Could you check a few things on this model? Use its own coordinates, in mm. Face numbers are marked on the shaded views. A direction names the side the tool comes from. Round coordinates to 2 decimals unless told otherwise and drop trailing zeros. Loops run counter-clockwise (first coordinate to the right, second up) from the corner with the lowest first, then second, coordinate; pieces in that order, holes last. Notation, with made-up numbers: (46, 69.5) -> (84, 69.5) arc R21 cw to (84, 92.5) -> close; hole circle Ø6 at (-9.75, 55). An arc over 180 degrees is marked (long way). Write each question's results on one line, items separated by ' | '.
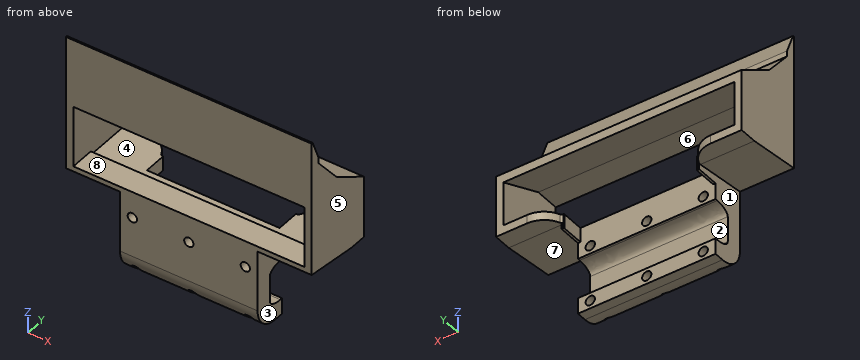
from build123d import *

# Parameters (mm, degrees)
RESSALTO_EXTRUS_O1_DEPTH = 30
CORTE_EXTRUS_O1_DEPTH    = 100
ESBO_O4_W                = 94
ESBO_O4_H                = 25
CORTE_EXTRUS_O2_DEPTH    = 10
ESBO_O5_W                = 94
ESBO_O5_H                = 18
CORTE_EXTRUS_O3_DEPTH    = 20
CORTE_EXTRUS_O7_START    = -3
CORTE_EXTRUS_O7_DEPTH    = 94
ESBO_O8_W                = 32
ESBO_O8_H                = 15
CORTE_EXTRUS_O8_DEPTH    = 56
ESBO_O9_W                = 16.5
ESBO_O9_H                = 8
CORTE_EXTRUS_O9_DEPTH    = 56
FILETE1_SIZE             = 3
FILETE1_SIZE_2           = 6
FILETE2_SIZE             = 3
FILETE2_SIZE_2           = 6
FILETE3_R                = 10
ESBO_O12_W               = 32
ESBO_O12_H               = 1
CORTE_EXTRUS_O12_DEPTH   = 68
CORTE_EXTRUS_O13_REACH   = 121.432
ESBO_O14_W               = 56
ESBO_O14_H               = 16
CORTE_EXTRUS_O14_DEPTH   = 138.840487586
ESBO_O16_R               = 1.9
CORTE_EXTRUS_O15_DEPTH   = 136.484316502
ESBO_O19_W               = 5.89
ESBO_O19_H               = 9.379485794
RESSALTO_EXTRUS_O4_DEPTH = 1
ESBO_O20_W               = 5.89
ESBO_O20_H               = 9.379485794
RESSALTO_EXTRUS_O5_DEPTH = 1
FILETE5_R                = 10
FILETE6_R                = 0.3
FILETE7_R                = 1
CORTE_EXTRUS_O17_DEPTH   = 22
CORTE_EXTRUS_O18_DEPTH   = 22
CORTE_EXTRUS_O19_DEPTH   = 124


with BuildPart() as part:
    # Esboço2 → Ressalto-extrusão1 (new body)
    with BuildSketch(Plane(origin=(0, 0, 0), x_dir=(1, 0, 0), z_dir=(0, 1, 0))):
        Polygon((0, 0), (0, 58), (22, 58), (22, 90), (78, 90), (78, 58), (100, 58), (100, 0), align=None)
    extrude(amount=RESSALTO_EXTRUS_O1_DEPTH)

    # Esboço3 → Corte-extrusão1 (cut)
    with BuildSketch(Plane(origin=(100, 0, 0), x_dir=(0, 0, -1), z_dir=(1, 0, 0))):
        Polygon((0, 0.6), (9.828405069, 4.570933406), (22.126818959, 14.890527965), (31.568264957, 30), (0, 30), align=None)
    extrude(amount=-CORTE_EXTRUS_O1_DEPTH, mode=Mode.SUBTRACT)

    # Esboço4 → Corte-extrusão2 (cut)
    with BuildSketch(Plane.XZ):
        with Locations((50, -40.5)):
            Rectangle(ESBO_O4_W, ESBO_O4_H)
    extrude(amount=-CORTE_EXTRUS_O2_DEPTH, mode=Mode.SUBTRACT)

    # Esboço5 → Corte-extrusão3 (cut)
    with BuildSketch(Plane(origin=(0, 30, 0), x_dir=(1, 0, 0), z_dir=(0, 1, 0))):
        with Locations((50, 45.5)):
            Rectangle(ESBO_O5_W, ESBO_O5_H)
    extrude(amount=-CORTE_EXTRUS_O3_DEPTH, mode=Mode.SUBTRACT)

    # Esboço7 → Corte-extrusão7 (cut)
    with BuildSketch(Plane(origin=(100, 0, 0), x_dir=(0, 0, -1), z_dir=(1, 0, 0)).offset(CORTE_EXTRUS_O7_START)):
        Polygon((28, 10), (36.5, 30), (36.5, 10), align=None)
    extrude(amount=-CORTE_EXTRUS_O7_DEPTH, mode=Mode.SUBTRACT)

    # Esboço8 → Corte-extrusão8 (cut)
    with BuildSketch(Plane(origin=(78, 0, 0), x_dir=(0, 0, -1), z_dir=(1, 0, 0))):
        with Locations((74, 22.5)):
            Rectangle(ESBO_O8_W, ESBO_O8_H)
    extrude(amount=-CORTE_EXTRUS_O8_DEPTH, mode=Mode.SUBTRACT)

    # Esboço9 → Corte-extrusão9 (cut)
    with BuildSketch(Plane(origin=(78, 0, 0), x_dir=(0, 0, -1), z_dir=(1, 0, 0))):
        with Locations((75.25, 11)):
            Rectangle(ESBO_O9_W, ESBO_O9_H)
    extrude(amount=-CORTE_EXTRUS_O9_DEPTH, mode=Mode.SUBTRACT)

    # Filete1
    # an asymmetric fillet: 6, 3 mm, written as the material it adds along each edge
    with BuildSketch(Plane(origin=(78, 7, -67), x_dir=(0, 0, -1), z_dir=(-1, 0, 0))) as filete1_piece_1:
        with BuildLine():
            Bezier((FILETE1_SIZE, 0), (0, 0), (0, -FILETE1_SIZE_2), weights=[1, 0.707106781, 1])
            Line((0, -FILETE1_SIZE_2), (0, 0))
            Line((0, 0), (FILETE1_SIZE, 0))
        make_face()
    extrude(amount=56)

    # Filete2
    # an asymmetric fillet: 6, 3 mm, written as the material it adds along each edge
    with BuildSketch(Plane(origin=(78, 7, -83.5), x_dir=(0, 0, 1), z_dir=(-1, 0, 0))) as filete2_piece_1:
        with BuildLine():
            Bezier((FILETE2_SIZE, 0), (0, 0), (0, FILETE2_SIZE_2), weights=[1, 0.707106781, 1])
            Line((0, FILETE2_SIZE_2), (0, 0))
            Line((0, 0), (FILETE2_SIZE, 0))
        make_face()
    extrude(amount=56)

    # Filete3
    filete3_edges = [part.edges().sort_by_distance(p)[0] for p in [
        (50, 0, -90),
    ]]
    fillet(filete3_edges, radius=FILETE3_R)

    # Esboço12 → Corte-extrusão12 (cut)
    with BuildSketch(Plane.ZY.offset(-22)):
        with Locations((-74, 14.5)):
            Rectangle(ESBO_O12_W, ESBO_O12_H)
    extrude(amount=-CORTE_EXTRUS_O12_DEPTH, mode=Mode.SUBTRACT)

    # Esboço14 → Corte-extrusão13 (cut, up to next)
    with BuildSketch(Plane(origin=(0, 0, -58), x_dir=(-1, 0, 0), z_dir=(0, 0, -1)), mode=Mode.PRIVATE) as corte_extrus_o13_sk1:
        with Locations((-50, 22)):
            Rectangle(ESBO_O14_W, ESBO_O14_H)
    corte_extrus_o13_tool1 = extrude(corte_extrus_o13_sk1.sketch, amount=-CORTE_EXTRUS_O13_REACH, mode=Mode.PRIVATE) & part.part
    add(corte_extrus_o13_tool1.solids().sort_by_distance((50, 22, -58))[0], mode=Mode.SUBTRACT)

    # Esboço15 → Corte-extrusão14 (cut, through all)
    with BuildSketch(Plane(origin=(100, 0, 0), x_dir=(0, 0, -1), z_dir=(1, 0, 0))):
        Polygon((9.048997211, 4.256032191), (10.048997211, 4.256032191), (10.048997211, 4.756032191), align=None)
    extrude(amount=-CORTE_EXTRUS_O14_DEPTH, mode=Mode.SUBTRACT)

    # Esboço16 → Corte-extrusão15 (cut, through all)
    with BuildSketch(Plane(origin=(0, 14, 0), x_dir=(1, 0, 0), z_dir=(0, 1, 0))):
        with Locations(Location((73, 86.75, 0), (0, 0, 270))):
            Circle(ESBO_O16_R)
        with Locations(Location((27, 86.75, 0), (0, 0, 270))):
            Circle(ESBO_O16_R)
        with Locations(Location((73, 63.75, 0), (0, 0, 90))):
            Circle(ESBO_O16_R)
        with Locations(Location((27, 63.75, 0), (0, 0, 90))):
            Circle(ESBO_O16_R)
        with Locations(Location((50, 86.75, 0), (0, 0, 270))):
            Circle(ESBO_O16_R)
        with Locations(Location((50, 63.75, 0), (0, 0, 90))):
            Circle(ESBO_O16_R)
    extrude(amount=-CORTE_EXTRUS_O15_DEPTH, mode=Mode.SUBTRACT)

    # Esboço19 → Ressalto-extrusão4 (add)
    with BuildSketch(Plane.ZY.offset(-78)):
        with Locations((-57.445, 18.689742897)):
            Rectangle(ESBO_O19_W, ESBO_O19_H)
    extrude(amount=RESSALTO_EXTRUS_O4_DEPTH)

    # Esboço20 → Ressalto-extrusão5 (add)
    with BuildSketch(Plane(origin=(22, 0, 0), x_dir=(0, 0, -1), z_dir=(1, 0, 0))):
        with Locations((57.445, 18.689742897)):
            Rectangle(ESBO_O20_W, ESBO_O20_H)
    extrude(amount=RESSALTO_EXTRUS_O5_DEPTH)

    # Filete5
    # the kernel refuses this fillet: 10 mm, written as the material it takes off along each edge
    with BuildSketch(Plane(origin=(22, 30, -81.529114381), x_dir=(0, -1, 0), z_dir=(0, 0, 1))) as filete5_piece_1_section:
        with BuildLine():
            CenterArc((10, -9.411645752), FILETE5_R, 109.75193963, 70.24806037)
            Line((0, -9.411645752), (0, 0))
            Line((0, 0), (6.620514206, 0))
        make_face()
    filete5_piece_1 = extrude(amount=50.558228762, mode=Mode.PRIVATE)
    filete5_piece_1 = split(filete5_piece_1, bisect_by=Plane(origin=(18.353344597, 35.581105786, -38.871969959), z_dir=(0, -0.39114064034485163, -0.9203309184584747)), keep=Keep.TOP, mode=Mode.PRIVATE)
    add(filete5_piece_1, mode=Mode.SUBTRACT)
    with BuildSketch(Plane(origin=(78, 30, -81.529114381), x_dir=(0, -1, 0), z_dir=(0, 0, 1))) as filete5_piece_2_section:
        with BuildLine():
            CenterArc((10, 9.411645752), FILETE5_R, 180, 70.24806037)
            Line((0, 9.411645752), (0, 0))
            Line((0, 0), (6.620514206, 0))
        make_face()
    filete5_piece_2 = extrude(amount=50.558228762, mode=Mode.PRIVATE)
    filete5_piece_2 = split(filete5_piece_2, bisect_by=Plane(origin=(81.646655403, 35.581105786, -38.871969959), z_dir=(0, -0.39114064034485163, -0.9203309184584747)), keep=Keep.TOP, mode=Mode.PRIVATE)
    add(filete5_piece_2, mode=Mode.SUBTRACT)

    # Filete6
    filete6_edges = [part.edges().sort_by_distance(p)[0] for p in [
        (77, 23.379485794, -57.445),
        (23, 23.379485794, -57.445),
    ]]
    fillet(filete6_edges, radius=FILETE6_R)

    # Filete7
    filete7_edges = [part.edges().sort_by_distance(p)[0] for p in [
        (78, 23.379485794, -56.25),
        (22, 23.379485794, -56.25),
    ]]
    fillet(filete7_edges, radius=FILETE7_R)

    # Esboço22 → Corte-extrusão17 (cut)
    with BuildSketch(Plane.ZY):
        Polygon((-58, 0), (-58, 22.70530007), (-55.105367164, 0), align=None)
    extrude(amount=-CORTE_EXTRUS_O17_DEPTH, mode=Mode.SUBTRACT)

    # Esboço23 → Corte-extrusão18 (cut)
    with BuildSketch(Plane(origin=(100, 0, 0), x_dir=(0, 0, -1), z_dir=(1, 0, 0))):
        Polygon((58, 0), (55.102867158, 0), (58, 22.71), align=None)
    extrude(amount=-CORTE_EXTRUS_O18_DEPTH, mode=Mode.SUBTRACT)

    # Esboço27 → Corte-extrusão19 (cut)
    with BuildSketch(Plane.ZY):
        Polygon((-31.568264957, 30), (-22.126818959, 14.890527965), (-10.048997211, 4.756032191), (-7.995032748, 3.989987748), (-10.691784821, 3.989987748), (-22.89093609, 14.226291078), (-32.747443361, 30), align=None)
    extrude(amount=-CORTE_EXTRUS_O19_DEPTH, mode=Mode.SUBTRACT)


solid = part.part
1) I want a section at B-B, the plane z = -49.5. Write out the boundary of the cut face in (x, y).
Model answer:
outline: (0, 0) -> (3, 0) -> (3, 30) -> (0, 30) -> close; (97, 0) -> (100, 0) -> (100, 30) -> (97, 30) -> close
2) For the marked faces 1, 2, 3 and 4, which set-ups out of +Z, -Z, +X, -X, +Y, -Y let a thin tool reach every point of the face, with its end or its side?
Model answer:
face 1: -Z, -X, -Y | face 2: +X, -X, +Y | face 3: -Z, +X, -Y | face 4: +Y
3) I need wall thicknesses on line 1 (X direction, y = 5, z = -63.75); line 2 (Z direction, x = 50, y = 6); line 3 (X direction, y = 4.5, z = -52). Which ranges of each line are inside material? Lowest first, please.
Model answer:
line 1: x = 22 to 25.1, 28.9 to 48.1, 51.9 to 71.1, 74.9 to 78 | line 2: z = -89.17 to -88.65, -84.85 to -65.65, -61.85 to -53, -28 to -13.09 | line 3: x = 0 to 3, 97 to 100
4) I want a section at A-A, the plane z = -63.75. Write out the boundary of the cut face in (x, y).
Model answer:
outline: (22, 0) -> (25.1, 0) -> (25.1, 14) -> (22, 14) -> close; (28.9, 0) -> (48.1, 0) -> (48.1, 14) -> (28.9, 14) -> close; (51.9, 0) -> (71.1, 0) -> (71.1, 14) -> (51.9, 14) -> close; (74.9, 0) -> (78, 0) -> (78, 14) -> (74.9, 14) -> close
5) If we mould it in two halves opening along Z, with no side actions, what happens to the marked faces 5, 6, 7 and 8? For each: released by +Z, released by -Z, zero draft, split by the parting line, or undercut.
Model answer:
face 5: zero draft | face 6: undercut | face 7: released by -Z | face 8: undercut
6) I want a section at D-D, the plane y = 21.5. Write out the boundary of the cut face in (x, z).
Model answer:
outline: (0, -57.85) -> (22, -57.85) -> (22, -60.39) -> (23, -60.39) -> (23, -54.5) -> (3, -54.5) -> (3, -32.89) -> (97, -32.89) -> (97, -54.5) -> (77, -54.5) -> (77, -60.39) -> (78, -60.39) -> (78, -57.85) -> (100, -57.85) -> (100, -27.44) -> (0, -27.44) -> close
7) I'm going to push flat-ended pins straight in: pin 1 (1.5 mm diameter, centred on x = 60, z = -9.5, fed in from +Y); pin 2 (3 mm diameter, centred on x = 53.5, y = 22.5, fed in from +Z); pin 3 (7 mm diameter, centred on x = 59.5, z = -88, fed in from +Y). Where does each tip first touch, or does it pass through?
Model answer:
pin 1: stops at y = 3.99 | pin 2: stops at z = -27.12 | pin 3: stops at y = 14
8) I want a section at C-C, the plane x = 79.5. Write out the boundary of the cut face in (y, z), plus the area to 3 significant figures.
Model answer:
outline: (0, -55.1) -> (22.71, -58) -> (26.12, -58) -> (26.12, -54.5) -> (10, -54.5) -> (10, -53) -> (0, -53) -> close; (0, -28) -> (10, -28) -> (30, -36.5) -> (30, -32.75) -> (14.23, -22.89) -> (3.99, -10.69) -> (3.99, -8.39) -> (0.6, 0) -> (0, 0) -> close | area: 374 mm2
